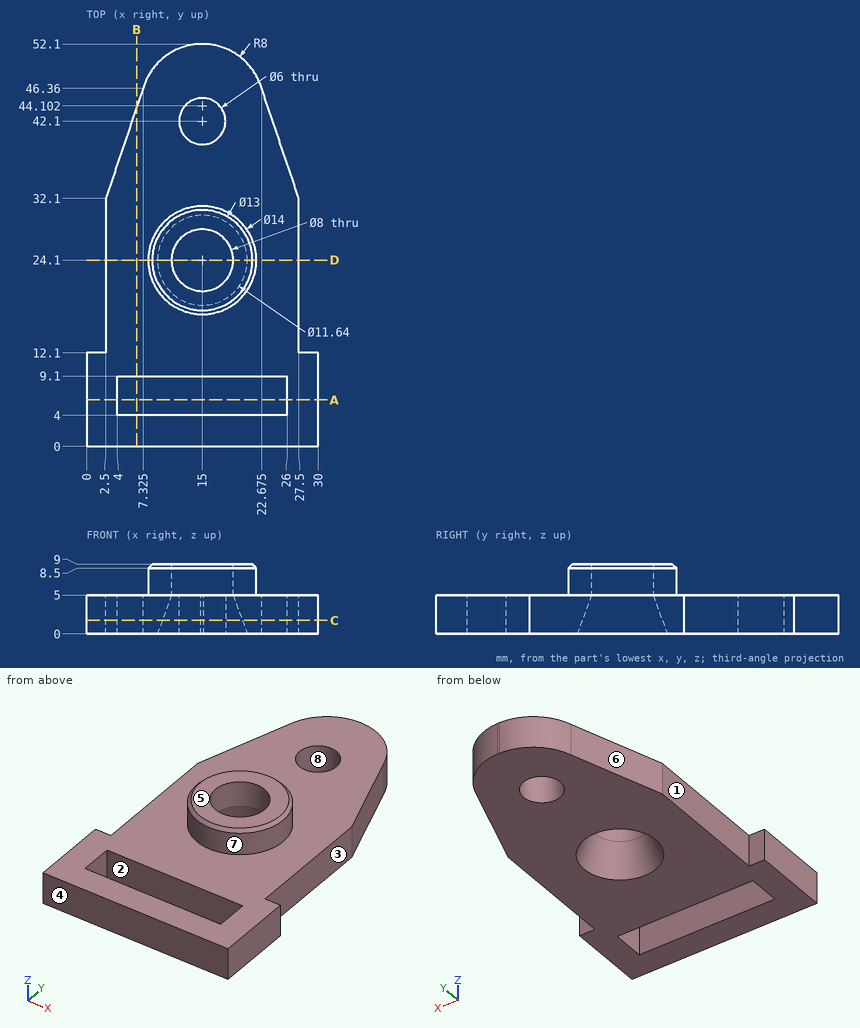
Can you work these out from the drawing? Everything is in mm from the part's minimum corner. A direction names the side the tool comes from. Round coordinates to 2 decimals unless told otherwise and drop trailing zeros. Loops run counter-clockwise (first coordinate to the right, second up) from the corner with the lowest first, then second, coordinate; pieces in that order, holes last. Notation, with made-up numbers: (64.25, 77) -> (110.25, 77) arc R18 cw to (110.25, 83) -> close; hole circle Ø3 at (-35.5, 33). An arc over 180 degrees is marked (long way). One line per question, with ' | ' between items.
(1) If we section it at C-C on z = 1.75: Count the separate pieces of the cut face and the enclosed holes in it, and give its area (3 significant figures).
Model answer:
separate pieces: 1 | enclosed holes: 3 | area: 991 mm^2
(2) If we section it at B-B on x = 6.5: List the corners of the cut face in (y, z) for me, and give its area (3 significant figures).
Model answer:
outline: (0, 0) -> (4, 0) -> (4, 5) -> (0, 5) -> close; (9.1, 0) -> (43.92, 0) -> (43.92, 5) -> (9.1, 5) -> close | area: 194 mm^2
(3) For pin 1 Ø1.2 at (x, z) = (29, 2) entering from +Y; pin 2 Ø1.5 at (y, z) = (17.5, 6.5) entering from -X (1 decimal); pin 3 Ø2.5 at (y, z) = (23, 2) entering from +X; pin 4 Ø9 at (x, y) = (18, 15) entering from +Z, each with a flat end and sliding along its axis, tell me the tip position at first contact or that it passes through.
Model answer:
pin 1: stops at y = 12.1 | pin 2: stops at x = 11.2 | pin 3: stops at x = 27.5 | pin 4: stops at z = 9
(4) If I drill on probe 1 along Y at (x, z) = (15, 8.25); probe 2 along Z at (x, y) = (25.5, 29); probe 3 along Y at (x, z) = (8.5, 0.5) (1 decimal), over which ranges is the centre line in solid material (lowest first)?
Model answer:
probe 1: y = 17.1 to 20.1, 28.1 to 31.1 | probe 2: z = 0 to 5 | probe 3: y = 0 to 4, 9.1 to 48.8
(5) If we section it at D-D on y = 24.1: List the corners of the cut face in (x, z) for me.
Model answer:
outline: (2.5, 0) -> (9.18, 0) -> (11, 5) -> (11, 9) -> (8.5, 9) -> (8, 8.5) -> (8, 5) -> (2.5, 5) -> close; (19, 5) -> (20.82, 0) -> (27.5, 0) -> (27.5, 5) -> (22, 5) -> (22, 8.5) -> (21.5, 9) -> (19, 9) -> close
(6) Thinking about a two-plate mould opening in Y: for the marked faces 5, 6, 7 and 8, which applies, released by +Y, released by -Y, zero draft, split by the parting line, or undercut?
Model answer:
face 5: zero draft | face 6: released by +Y | face 7: split by the parting line | face 8: undercut
(7) If we section it at A-A on y = 6: List the corners of the cut face in (x, z) for me.
Model answer:
outline: (0, 0) -> (4, 0) -> (4, 5) -> (0, 5) -> close; (26, 0) -> (30, 0) -> (30, 5) -> (26, 5) -> close
(8) For the marked faces 1, 2, 3 and 4, which set-ups out of +Z, -Z, +X, -X, +Y, -Y let a thin tool reach every point of the face, with its end or its side?
Model answer:
face 1: +Z, -Z, -X, +Y | face 2: +Z, -Z | face 3: +Z, -Z, +X, +Y | face 4: +Z, -Z, +X, -X, -Y
